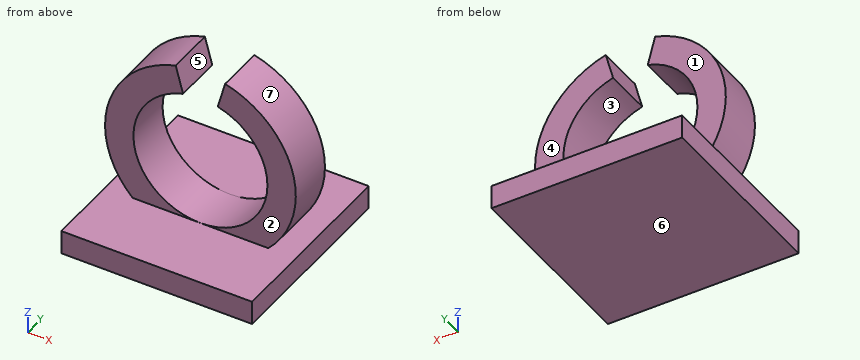
from build123d import *

# Parameters (mm, degrees)
F0_W     = 20
F0_H     = 20
F1_DEPTH = 2.5
F3_DEPTH = 1.5
F4_DEPTH = 2.5
F5_DEPTH = 2


with BuildPart() as f1:
    # F0 (on Top) → F1 (new body)
    with BuildSketch(Plane.XY):
        Rectangle(F0_W, F0_H)
    extrude(amount=F1_DEPTH)

    # F2 (on Front) → F3 (join, symmetric)
    with BuildSketch(Plane.XZ):
        with BuildLine():
            Line((-1.818204, 16.310629), (-2.58819, 19.184258))
            ThreePointArc((-2.58819, 19.184258), (-9.997161, 9.76325), (-3.045386, 0))
            Line((-3.045386, 0), (3.045386, 0))
            ThreePointArc((3.045386, 0), (9.997161, 9.76325), (2.58819, 19.184258))
            Line((2.58819, 19.184258), (1.818204, 16.310629))
            ThreePointArc((1.818204, 16.310629), (0, 2.5), (-1.818204, 16.310629))
        make_face()
    extrude(amount=F3_DEPTH, both=True)

    # F2 (on Front) → F4 (join, symmetric)
    with BuildSketch(Plane.XZ):
        with BuildLine():
            Line((-1.818204, 16.310629), (-2.58819, 19.184258))
            ThreePointArc((-2.58819, 19.184258), (-9.997161, 9.76325), (-3.045386, 0))
            Line((-3.045386, 0), (3.045386, 0))
            ThreePointArc((3.045386, 0), (9.997161, 9.76325), (2.58819, 19.184258))
            Line((2.58819, 19.184258), (1.818204, 16.310629))
            ThreePointArc((1.818204, 16.310629), (0, 2.5), (-1.818204, 16.310629))
        make_face()
    extrude(amount=F4_DEPTH, both=True)

    # F2 (on Front) → F5 (join, symmetric)
    with BuildSketch(Plane.XZ):
        with BuildLine():
            Line((-1.818204, 16.310629), (-2.58819, 19.184258))
            ThreePointArc((-2.58819, 19.184258), (-9.997161, 9.76325), (-3.045386, 0))
            Line((-3.045386, 0), (3.045386, 0))
            ThreePointArc((3.045386, 0), (9.997161, 9.76325), (2.58819, 19.184258))
            Line((2.58819, 19.184258), (1.818204, 16.310629))
            ThreePointArc((1.818204, 16.310629), (0, 2.5), (-1.818204, 16.310629))
        make_face()
    extrude(amount=F5_DEPTH, both=True)


solid = f1.part
For this review, take the finished solid that the model builds, in its own axes (mm). Face numbers are marked on the shaded views. A direction names the side the tool comes from. Coordinates: 2 decimals unless noted, no trailing zeros. Order: outer loops, then holes, each group sorted by start corner. A loop starts at its lowest first (then second) coordinate and runs counter-clockwise, first axis right, second up. Notation, with made-up numbers: (-32.75, 78) -> (-27.75, 78) arc R12 cw to (-27.75, 93) -> close; hole circle Ø3 at (-24.75, 10). An arc over 180 degrees is marked (long way). Return JSON: item names as keys, results as strings.
1. For line 1 (Y direction, x = 8.25, z = 13.5); line 2 (Z direction, x = 4.75, y = 7.25); line 3 (X direction, y = -2.25, z = 14.5), list the stretches that pass through material, from the lowest coordinate up. Write a range as from..to.
Answer block:
{"line 1": "-2.5..2.5", "line 2": "0..2.5", "line 3": "-8.67..-4.96, 4.96..8.67"}
2. The part is to be moulded in two halves that separate along Z. For the marked faces 4, 5, 6 and 7, say which applies: +Z half, -Z half, draft (parallel to the pull), parting line (faces both ways), or undercut.
Answer block:
{"face 4": "draft", "face 5": "+Z half", "face 6": "-Z half", "face 7": "undercut"}
3. We need section B-B on x = 5.5. Write out the cut boundary in (y, z), and give its area (3 significant figures).
Answer block:
{"outline": "(-10, 0) -> (10, 0) -> (10, 2.5) -> (2.5, 2.5) -> (2.5, 5.15) -> (-2.5, 5.15) -> (-2.5, 2.5) -> (-10, 2.5) -> close; (-2.5, 13.9) -> (2.5, 13.9) -> (2.5, 17.88) -> (-2.5, 17.88) -> close", "area": "83.2 mm²"}
4. We need section A-A on z = 15.5. Write out the cut boundary in (x, y).
Answer block:
{"outline": "(-8.02, -2.5) -> (-3.69, -2.5) -> (-3.69, 2.5) -> (-8.02, 2.5) -> close; (3.69, -2.5) -> (8.02, -2.5) -> (8.02, 2.5) -> (3.69, 2.5) -> close"}
5. Machinability: for the marked faces 1, 2 and 3, which of the approach directions +Z, -Z, +X, -X, +Y, -Y give a long, thin tool a straight path to every point of the face, cutting with its end or side? Answer none if there is none.
Answer block:
{"face 1": "+Z, +X, -X, +Y", "face 2": "+Z, +X, -X, -Y", "face 3": "+Y, -Y"}
6. We need section D-D on z = 10.75. Write out the cut boundary in (x, y), and give its area (3 significant figures).
Answer block:
{"outline": "(-9.92, -2.5) -> (-6.92, -2.5) -> (-6.92, 2.5) -> (-9.92, 2.5) -> close; (6.92, -2.5) -> (9.92, -2.5) -> (9.92, 2.5) -> (6.92, 2.5) -> close", "area": "30.1 mm²"}
7. We need section C-C on y = -2. Write out the cut boundary in (x, z) (3 decimals).
Answer block:
{"outline": "(-10, 0) -> (10, 0) -> (10, 2.5) -> (7.117, 2.5) arc R10 ccw to (2.588, 19.184) -> (1.818, 16.311) arc R7.025 cw (long way) to (-1.818, 16.311) -> (-2.588, 19.184) arc R10 ccw to (-7.117, 2.5) -> (-10, 2.5) -> close"}
8. For pin 1 Ø5 at (x, z) = (7, 9.5) entering from -Y; pin 2 Ø5 at (x, z) = (-6.5, 11.5) entering from +Y; pin 3 Ø1 at (y, z) = (7, 3.5) entering from -X; pin 4 Ø6 at (y, z) = (0.5, 11) entering from -X, all flat-tipped, find the tip position at first contact; note any pin that passes through.
Answer block:
{"pin 1": "y = -2.5", "pin 2": "y = 2.5", "pin 3": "through", "pin 4": "x = -10"}
